from build123d import *

# Parameters (mm, degrees)
SKETCH1_R           = 40
BOSS_EXTRUDE1_DEPTH = 20
SKETCH2_W           = 91.95154217
SKETCH2_H           = 92.440305864
SKETCH2_W_2         = 78
SKETCH2_H_2         = 78
CUT_EXTRUDE3_DEPTH  = 61
SKETCH3_R           = 2.5
CUT_EXTRUDE5_DEPTH  = 59.668560575
SKETCH5_R           = 3
CUT_EXTRUDE6_DEPTH  = 90.470665584
SKETCH6_R           = 3
CUT_EXTRUDE7_DEPTH  = 90.470665584
SKETCH7_R           = 20
CUT_EXTRUDE8_DEPTH  = 59.668560575
CHAMFER1_SIZE       = 2
SKETCH8_R           = 3
CUT_EXTRUDE9_DEPTH  = 5


with BuildPart() as part:
    # Sketch1 → Boss-Extrude1 (new body)
    with BuildSketch(Plane.XY):
        Circle(SKETCH1_R)
    extrude(amount=BOSS_EXTRUDE1_DEPTH)

    # Sketch2 → Cut-Extrude3 (cut, through all)
    with BuildSketch(Plane(origin=(0, 0, 0), x_dir=(-1, 0, 0), z_dir=(0, 0, -1))):
        Rectangle(SKETCH2_W, SKETCH2_H)
        Rectangle(SKETCH2_W_2, SKETCH2_H_2, mode=Mode.SUBTRACT)
    extrude(amount=-CUT_EXTRUDE3_DEPTH, mode=Mode.SUBTRACT)

    # Sketch3 → Cut-Extrude5 (cut, through all)
    with BuildSketch(Plane(origin=(0, 0, 0), x_dir=(-1, 0, 0), z_dir=(0, 0, -1))):
        with Locations((21.213203436, 21.213203436)):
            Circle(SKETCH3_R)
        with Locations((21.213203436, -21.786796564)):
            Circle(SKETCH3_R)
        with Locations((-21.786796564, -21.786796564)):
            Circle(SKETCH3_R)
        with Locations((-21.786796564, 21.213203436)):
            Circle(SKETCH3_R)
    extrude(amount=-CUT_EXTRUDE5_DEPTH, mode=Mode.SUBTRACT)

    # Sketch5 → Cut-Extrude6 (cut, through all)
    with BuildSketch(Plane(origin=(39, 0, 0), x_dir=(0, 0, -1), z_dir=(1, 0, 0))):
        with Locations((-10, 0)):
            Circle(SKETCH5_R)
    extrude(amount=-CUT_EXTRUDE6_DEPTH, mode=Mode.SUBTRACT)

    # Sketch6 → Cut-Extrude7 (cut, through all)
    with BuildSketch(Plane.XZ.offset(39)):
        with Locations((0, 10)):
            Circle(SKETCH6_R)
    extrude(amount=-CUT_EXTRUDE7_DEPTH, mode=Mode.SUBTRACT)

    # Sketch7 → Cut-Extrude8 (cut, through all)
    with BuildSketch(Plane(origin=(0, 0, 0), x_dir=(-1, 0, 0), z_dir=(0, 0, -1))):
        Circle(SKETCH7_R)
    extrude(amount=-CUT_EXTRUDE8_DEPTH, mode=Mode.SUBTRACT)

    # Fillet2: read off the stored shape, not the designer's step
    # Fillet2 outline → Fillet2 (revolve, cut)
    with BuildSketch(Plane.XZ):
        with BuildLine():
            ThreePointArc((37, 20), (39.121320386, 19.121320302), (40, 16.999999881))
            Line((40, 16.999999881), (40, 20))
            Line((40, 20), (37, 20))
        make_face()
        with BuildLine():
            Line((40, 0), (40, 3.000000119))
            ThreePointArc((40, 3.000000119), (39.121320386, 0.878679698), (37, 0))
            Line((37, 0), (40, 0))
        make_face()
    revolve(axis=Axis((0, 0, 0), (0, 0, 1)), mode=Mode.SUBTRACT)

    # Chamfer1
    chamfer1_edges = [part.edges().sort_by_distance(p)[0] for p in [
        (20, 0, 20),
        (20, 0, 0),
    ]]
    chamfer(chamfer1_edges, length=CHAMFER1_SIZE)

    # Sketch8 → Cut-Extrude9 (cut)
    with BuildSketch(Plane(origin=(150.63801623, 159.049980591, 20), x_dir=(0, -1, 0), z_dir=(0, 0, 1))):
        with Locations(Location((192.049980649, -156.798016257, 0), (0, 0, 90))):
            Circle(SKETCH8_R)
        with Locations(Location((126.049980533, -156.798016257, 0), (0, 0, 270))):
            Circle(SKETCH8_R)
    extrude(amount=-CUT_EXTRUDE9_DEPTH, mode=Mode.SUBTRACT)


solid = part.part
The listing builds one solid part. Answer for the finished solid, in the listing's coordinates (mm). A direction names the side the tool comes from. Coordinates: 2 decimals unless noted, no trailing zeros. Write each loop counter-clockwise with the first axis right and the second up, starting at its lowest first coordinate (ties: lowest second). Pieces come first, ordered by that corner, then holes. Notation, with made-up numbers: (64.25, 85) - (83.25, 85) arc R24 cw to (83.25, 118) - close; hole circle Ø3 at (-38.75, 2.5). An arc over 180 degrees is marked (long way). Return JSON: item names as keys, results as strings.
1. For a pull along X with two mould halves and no side action, classify faces 1 (the face through (28.061, -28.506, 9.902)), 2 (the face through (-3, 29, 10)), 3 (the face through (-29.3, -1.8, 12.4)) as +X half, -X half, draft (parallel to the pull), parting line (faces both ways), or undercut.
Final values:
{"face 1": "+X half", "face 2": "undercut", "face 3": "draft"}
2. The part is cut by section A-A on y = 0. Determine the outline of the cut face in (x, z).
Final values:
{"outline": "(-39, 0.76) arc R3 ccw to (-37, 0) - (-22, 0) - (-20, 2) - (-20, 7) - (-39, 7) - close; (-39, 13) - (-20, 13) - (-20, 18) - (-22, 20) - (-37, 20) arc R3 ccw to (-39, 19.24) - close; (20, 2) - (22, 0) - (37, 0) arc R3 ccw to (39, 0.76) - (39, 7) - (20, 7) - close; (20, 13) - (39, 13) - (39, 19.24) arc R3 ccw to (37, 20) - (22, 20) - (20, 18) - close"}
3. Which of the six approach directions +Z, -Z, +X, -X, +Y, -Y give full straight-line access (tool end or side, diameter ignored) to faces 4 (the face through (-6, -33, 15)), 5 (the face through (-28.061, 28.506, 9.902))?
Final values:
{"face 4": "+Z", "face 5": "+Z, -Z, -X, +Y"}
4. The part is cut by section C-C on z = 5. Determine the outline of the cut face in (x, y).
Final values:
{"outline": "(-39, -8.89) arc R40 ccw to (-8.89, -39) - (8.89, -39) arc R40 ccw to (39, -8.89) - (39, 8.89) arc R40 ccw to (8.89, 39) - (-8.89, 39) arc R40 ccw to (-39, 8.89) - close; hole circle Ø5 at (-21.21, -21.79); hole circle Ø5 at (-21.21, 21.21); hole circle Ø40 at (0, 0); hole circle Ø5 at (21.79, -21.79); hole circle Ø5 at (21.79, 21.21)"}
5. Each of these flat-tipped pins is pushed along its axis until it touches: pin 1 Ø1.5 at (x, y) = (-9, 20) entering from +Z; pin 2 Ø3 at (x, z) = (24, 15.5) entering from -Y; pin 3 Ø5 at (y, z) = (0, 10) entering from +X; pin 4 Ø3.5 at (x, y) = (-6.16, 33) entering from +Z. Where does it stop, or does it pass through?
Final values:
{"pin 1": "z = 20", "pin 2": "y = -33.07", "pin 3": "through", "pin 4": "z = 15"}
6. Consider line 1 along Z through (x, y) = (0, 31.5); line 2 along Y through (x, z) = (-3, 4.75); line 3 along X through (y, z) = (-22, 9.5). Determine where each line is inside the solid, lowest interval first.
Final values:
{"line 1": "0 to 7, 13 to 20", "line 2": "-39 to -19.77, 19.77 to 39", "line 3": "-33.41 to -23.7, -18.72 to -2.96, 2.96 to 19.3, 24.28 to 33.41"}
